Can you work these out from the model? Positions are in its coordinate system, mm. A direction names the side the tool comes from. Coordinates: 2 decimals unless noted, no trailing zeros. Write each loop counter-clockwise with the first axis right and the second up, starting at its lowest first coordinate (ties: lowest second). Pieces come first, ordered by that corner, then holes. Notation, with made-up numbers: (-11, 28.25) -> (18, 28.25) arc R7 cw to (18, 41.25) -> close; hole circle Ø11 at (-4.5, 3). An arc over 180 degrees is marked (long way). Use one line per item in the form item = value.
```python
from build123d import *

# Parameters (mm, degrees)
SKETCH4_W           = 95
SKETCH4_H           = 45.00899887
SKETCH4_R           = 1.54999944
BOSS_EXTRUDE6_DEPTH = 3


with BuildPart() as part:
    # Sketch4 → Boss-Extrude6 (new body)
    with BuildSketch(Plane.XY):
        with Locations((8.24074008, 34.620274583)):
            Rectangle(SKETCH4_W, SKETCH4_H)
        with Locations((42.74074118, 54.124774018)):
            Circle(SKETCH4_R, mode=Mode.SUBTRACT)
        with Locations((8.24073906, 15.115774228)):
            Circle(SKETCH4_R, mode=Mode.SUBTRACT)
        with Locations((-36.25926084, 54.124774018)):
            Circle(SKETCH4_R, mode=Mode.SUBTRACT)
        with BuildLine():
            Line((52.04074008, 55.624774018), (52.24074008, 55.624774018))
            ThreePointArc((52.24074008, 55.624774018), (53.654953642, 55.038987581), (54.24074008, 53.624774018))
            Line((54.24074008, 53.624774018), (54.24074008, 15.615775148))
            ThreePointArc((54.24074008, 15.615775148), (53.654953642, 14.201561585), (52.24074008, 13.615775148))
            Line((52.24074008, 13.615775148), (52.04074008, 13.615775148))
            ThreePointArc((52.04074008, 13.615775148), (50.626526517, 14.201561585), (50.04074008, 15.615775148))
            Line((50.04074008, 15.615775148), (50.04074008, 53.624774018))
            ThreePointArc((50.04074008, 53.624774018), (50.626526517, 55.038987581), (52.04074008, 55.624774018))
        make_face(mode=Mode.SUBTRACT)
        with BuildLine():
            Line((14.14745222, 50.977241122), (-27.788451431, 51.033818491))
            ThreePointArc((-27.788451431, 51.033818491), (-30.220596767, 53.472535297), (-27.781879961, 55.904680633))
            Line((-27.781879961, 55.904680633), (14.15402369, 55.848103264))
            ThreePointArc((14.15402369, 55.848103264), (16.586169026, 53.409386458), (14.14745222, 50.977241122))
        make_face(mode=Mode.SUBTRACT)
    extrude(amount=BOSS_EXTRUDE6_DEPTH)


solid = part.part
```
Q1. Will this pin go through, and if not, where does the flat tip stop? pin 1 (5 mm diameter, centred on x = -10, y = 26.5, fed in from -Z).
Return value:
pin_1 = 0
Q2. Suppose I cut it at B-B (x = -20). Write out the boundary of the cut face in (y, z), then the cut area to 3 significant figures.
Return value:
outline = (12.12, 0) -> (51.02, 0) -> (51.02, 3) -> (12.12, 3) -> close; (55.89, 0) -> (57.12, 0) -> (57.12, 3) -> (55.89, 3) -> close
area = 120 mm2
Q3. Suppose I cut it at C-C (z = 1.05). Write out the boundary of the cut face in (x, y).
Return value:
outline = (-39.26, 12.12) -> (55.74, 12.12) -> (55.74, 57.12) -> (-39.26, 57.12) -> close; hole circle Ø3.1 at (-36.26, 54.12); hole (-27.79, 51.03) -> (14.15, 50.98) arc R2.44 ccw to (14.15, 55.85) -> (-27.78, 55.9) arc R2.44 ccw to start; hole circle Ø3.1 at (8.24, 15.12); hole circle Ø3.1 at (42.74, 54.12); hole (50.04, 15.62) arc R2 ccw to (52.04, 13.62) -> (52.24, 13.62) arc R2 ccw to (54.24, 15.62) -> (54.24, 53.62) arc R2 ccw to (52.24, 55.62) -> (52.04, 55.62) arc R2 ccw to (50.04, 53.62) -> close
Q4. If I drill on line 1 (X direction, y = 39, z = 0.45); line 2 (Y direction, x = -24.5, z = 2.15); line 3 (X direction, y = 16.5, z = 1.35), over which ranges is the centre line in solid material (lowest first)? Write a range as from..to.
Return value:
line_1 = -39.26..50.04, 54.24..55.74
line_2 = 12.12..51.03, 55.9..57.12
line_3 = -39.26..7.54, 8.94..50.04, 54.24..55.74
Q5. Thinking about a two-plate mould opening in X: for faces 1 (the flat face through (55.741, 34, 1)), 2 (the flat face through (8, 35, 3)), 3 (the flat face through (-39.259, 34, 1)), 4 (the cylindrical face through (43.46, 52.75, 1.48)), which applies, released by +X, released by -X, zero draft, split by the parting line, or undercut?
Return value:
face_1 = released by +X
face_2 = zero draft
face_3 = released by -X
face_4 = undercut
Q6. For faces 5 (the flat face through (8, 12.116, 1)), 6 (the cylindrical face through (53.67, 14.217, 1.479)), which set-ups out of +Z, -Z, +X, -X, +Y, -Y let a thin tool reach every point of the face, with its end or its side?
Return value:
face_5 = +Z, -Z, +X, -X, -Y
face_6 = +Z, -Z
Q7. Suppose I cut it at A-A (y = 48). Write out the boundary of the cut face in (x, z).
Return value:
outline = (-39.26, 0) -> (50.04, 0) -> (50.04, 3) -> (-39.26, 3) -> close; (54.24, 0) -> (55.74, 0) -> (55.74, 3) -> (54.24, 3) -> close
